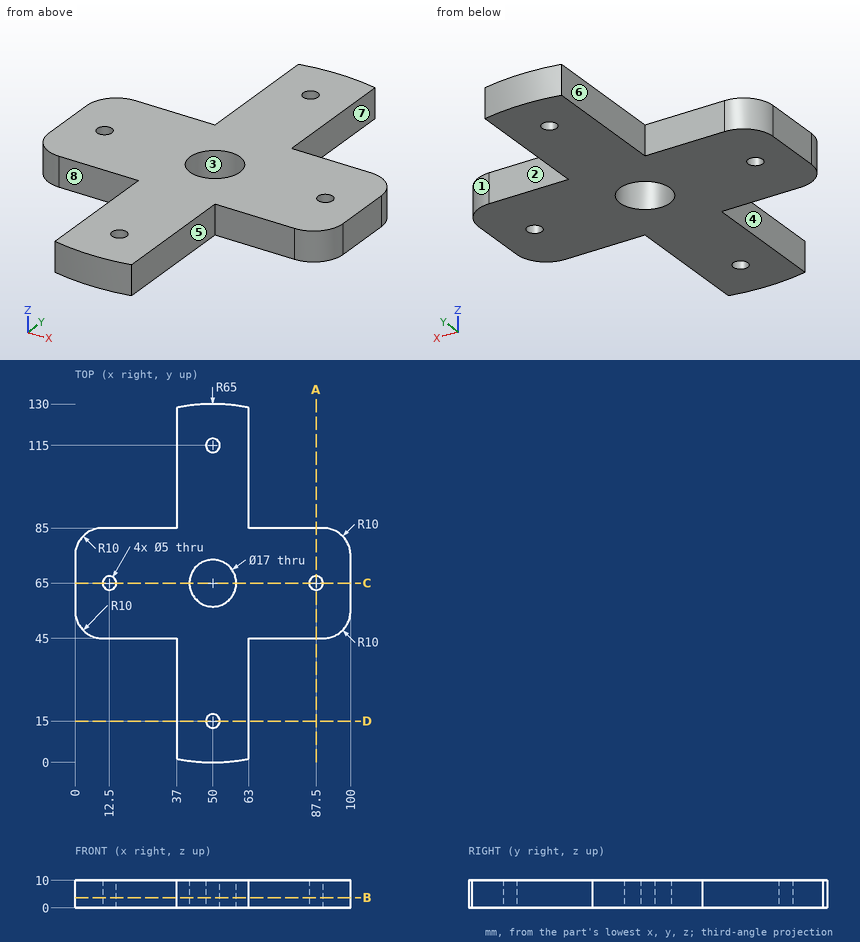
Print and shaded views of the part. All mm, measured from the part's lowest x, y and z. A direction names the side the tool comes from. Coordinates: 2 decimals unless noted, no trailing zeros. Write each loop counter-clockwise with the first axis right and the second up, starting at its lowest first coordinate (ties: lowest second). Pieces come first, ordered by that corner, then holes. Notation, with made-up numbers: M 33.5,-24 L 81.5,-24 A16 cw 81.5,-13 Z; hole C -13.5,59 d11. An arc over 180 degrees is marked long. Return JSON: item names as keys, results as strings.
1. Saw through at C-C, the plane y = 65. Write the cut outline in (x, z), then the cut area to 3 significant figures.
Determined:
{"outline": "M 0,0 L 10,0 L 10,10 L 0,10 Z; M 15,0 L 41.5,0 L 41.5,10 L 15,10 Z; M 58.5,0 L 85,0 L 85,10 L 58.5,10 Z; M 90,0 L 100,0 L 100,10 L 90,10 Z", "area": "730 mm²"}
2. Flat gauge pins, fed straight in: pin 1 Ø5 at (x, z) = (82, 3) entering from +Y; pin 2 Ø5 at (y, z) = (29, 5) entering from -X; pin 3 Ø5 at (x, z) = (39.5, 7.5) entering from -Y; pin 4 Ø10 at (x, y) = (50, 65) entering from +Z. Where does each tip first touch, or does it go through?
Determined:
{"pin 1": "y = 85", "pin 2": "x = 37", "pin 3": "y = 0.49", "pin 4": "through"}
3. Probe L1, parallel to Y at x = 50, z = 6; L2, parallel to Y at x = 12.5, z = 8; L3, parallel to Y at x = 30, z = 3.5. List the from-to ranges inside material, lowest first.
Determined:
{"L1": "0 to 12.5, 17.5 to 56.5, 73.5 to 112.5, 117.5 to 130", "L2": "45 to 62.5, 67.5 to 85", "L3": "45 to 85"}
4. Saw through at A-A, the plane x = 87.5. Write the cut outline in (y, z), then the cut area to 3 significant figures.
Determined:
{"outline": "M 45,0 L 62.5,0 L 62.5,10 L 45,10 Z; M 67.5,0 L 85,0 L 85,10 L 67.5,10 Z", "area": "350 mm²"}
5. Pull direction X, two halves, no side cores. Call the marked faces 1, 2, 3 and 4: pulls with the +X half, pulls with the -X half, needs draft (parallel to the pull), parting line crosses it, or undercut.
Determined:
{"face 1": "pulls with the +X half", "face 2": "needs draft", "face 3": "undercut", "face 4": "pulls with the -X half"}
6. Saw through at D-D, the plane y = 15. Write the cut outline in (x, z), then the cut area to 3 significant figures.
Determined:
{"outline": "M 37,0 L 47.5,0 L 47.5,10 L 37,10 Z; M 52.5,0 L 63,0 L 63,10 L 52.5,10 Z", "area": "210 mm²"}
7. Saw through at B-B, the plane z = 3.75. Write the cut outline in (x, y), then the cut area to 3 significant figures.
Determined:
{"outline": "M 0,55 A10 ccw 10,45 L 37,45 L 37,1.31 A65 ccw 63,1.31 L 63,45 L 90,45 A10 ccw 100,55 L 100,75 A10 ccw 90,85 L 63,85 L 63,128.69 A65 ccw 37,128.69 L 37,85 L 10,85 A10 ccw 0,75 Z; hole C 12.5,65 d5; hole C 50,65 d17; hole C 50,15 d5; hole C 50,115 d5; hole C 87.5,65 d5", "area": "5,930 mm²"}
8. 3-axis set-ups, long thin cutter, end or side, ignore diameter. For the marked faces 5, 6, 7 and 8: which of +Z, -Z, +X, -X, +Y, -Y reach the whole face in a straight line?
Determined:
{"face 5": "+Z, -Z, +X, -Y", "face 6": "+Z, -Z, -X, +Y", "face 7": "+Z, -Z, +X, +Y", "face 8": "+Z, -Z, -X, -Y"}
